Job drawing, mm, ordinate dimensions from the low corner. One solid piece. A direction names the side the tool comes from. Give positions to 0.01 mm unless a question says otherwise; leave off trailing zeros. Order: outer loops, then holes, each group sorted by start corner. A loop starts at its lowest first (then second) coordinate and runs counter-clockwise, first axis right, second up. Notation, with made-up numbers: (33.5, 2.25) -> (70.5, 2.25) arc R14 ccw to (70.5, 21.25) -> close; hole circle Ø3 at (70, 11.25). An arc over 180 degrees is marked (long way). Use CSV: the item, a comma, the result in double quotes. Start each with the question number.
1. Pull direction X, two halves, no side cores. Call the marked faces 3, 4, 5 and 6: released by +X, released by -X, zero draft, split by the parting line, or undercut.
2. Drop flat-ended pins along their axis: pin 1 (0.7 mm diameter, centred on x = 21.5, y = 5.5, fed in from -Z); pin 2 (0.7 mm diameter, centred on y = 2.5, z = 5.5, fed in from -X); pin 3 (1 mm diameter, centred on x = 15, z = 2.5, fed in from -Y); pin 4 (1.6 mm diameter, centred on y = 5, z = 5.5, fed in from +X). Give the stop position or say it passes through.
3. Cut at B-B on z = 3.25. List the corners of the cut face in (x, y), then the cut area to 3 significant figures.
4. Cut at A-A on x = 18.5. List the corners of the cut face in (y, z), then the cut area to 3 significant figures.
5. 3-axis set-ups, long thin cutter, end or side, ignore diameter. For the marked faces 1 and 2: which of +Z, -Z, +X, -X, +Y, -Y reach the whole face in a straight line?
6. Cut at C-C on y = 3.95. Give the number of separate pieces and of enclosed holes in the cut face, then the cut area to 3 significant figures.
7. Wall check: line 1 (X direction, y = 3.95, z = 5.3); line 2 (Z direction, x = 17.75, y = 3.25); line 3 (Y direction, x = 11.7, z = 7.1). Give the ranges that are in metal, low to high. Write a range as from..to.
8. Cut at D-D on z = 0.5. List the corners of the cut face in (x, y).
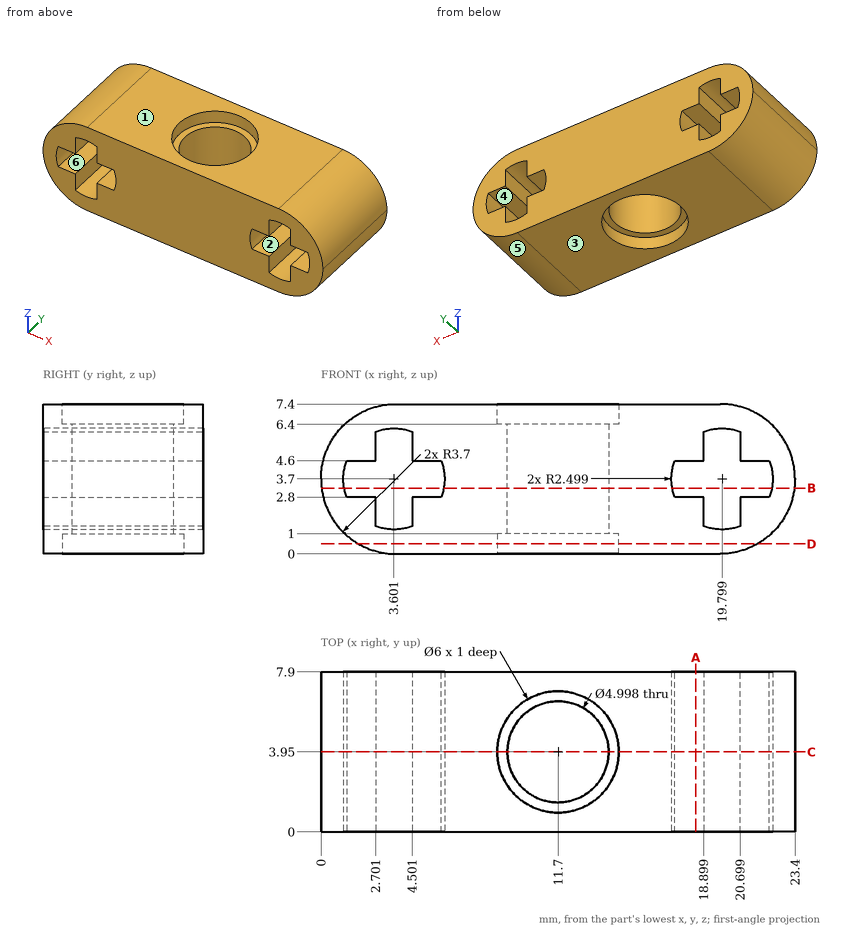
Verdict:
1,face 3,"zero draft"
1,face 4,"undercut"
1,face 5,"released by +X"
1,face 6,"undercut"
2,pin 1,"z = 0.3"
2,pin 2,"x = 0.3"
2,pin 3,"y = 0"
2,pin 4,"x = 23.26"
3,outline,"(0.03, 0) -> (1.14, 0) -> (1.14, 7.9) -> (0.03, 7.9) -> close; (6.06, 0) -> (17.34, 0) -> (17.34, 7.9) -> (6.06, 7.9) -> close; (22.26, 0) -> (23.37, 0) -> (23.37, 7.9) -> (22.26, 7.9) -> close; hole circle Ø5 at (11.7, 3.95)"
3,area,"87.1 mm^2"
4,outline,"(0, 0) -> (7.9, 0) -> (7.9, 2.8) -> (0, 2.8) -> close; (0, 4.6) -> (7.9, 4.6) -> (7.9, 7.4) -> (0, 7.4) -> close"
4,area,"44.2 mm^2"
5,face 1,"+Z, +X, -X, +Y, -Y"
5,face 2,"+Y, -Y"
6,separate pieces,"2"
6,enclosed holes,"2"
6,area,"93.7 mm^2"
7,line 1,"0.36..2.7, 4.5..9.2, 14.2..18.9, 20.7..23.04"
7,line 2,"0..2.8, 4.6..7.4"
7,line 3,"0..0.95, 6.95..7.9"
8,outline,"(1.84, 0) -> (21.56, 0) -> (21.56, 7.9) -> (1.84, 7.9) -> close; hole circle Ø6 at (11.7, 3.95)"
